Part model, mm, in its own coordinate system. Round coordinates to 2 decimals unless told otherwise and drop trailing zeros. Loops run counter-clockwise (first coordinate to the right, second up) from the corner with the lowest first, then second, coordinate; pieces in that order, holes last. Notation, with made-up numbers: (54.25, 18.5) -> (101.25, 18.5) arc R14 ccw to (101.25, 45.5) -> close; hole circle Ø8 at (57, -28.5). An arc over 180 degrees is marked (long way). Use a Markdown table: item, result. Add a question column.
Item 1: Flat gauge pin, fed straight in: pin 1 (15 mm diameter, centred on x = 437.11, z = -80.34, fed in from +Y) (1 decimal). Where does the tip first touch, or does it go through?
Item 2: Probe line 1 (X direction, y = 15.75, z = -48.5); line 2 (X direction, y = 4.5, z = -76.5). List the from-to ranges inside material, lowest first. Write a range as [from, to].
Item 3: Cut at C-C, the plane z = -82.5. List the corners of the cut face in (x, y), plus the area to 3 significant figures.
Item 4: Cut at B-B, the plane y = 10.5. List the corners of the cut face in (x, z), plus the area to 3 significant figures.
Item 5: Cut at A-A, the plane z = -37.5. List the corners of the cut face in (x, y).
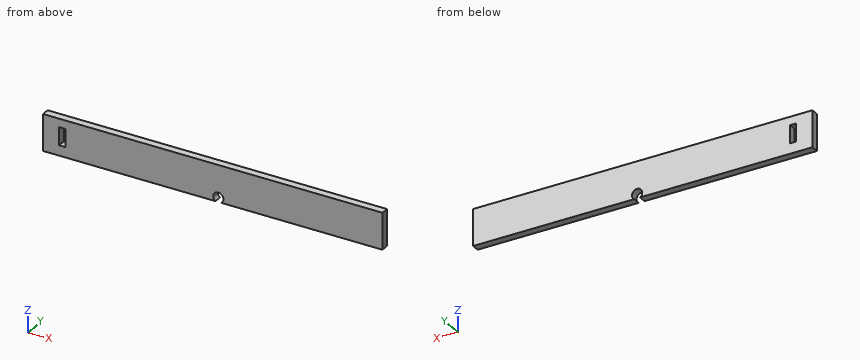
```python
from build123d import *

# Parameters (mm, degrees)
SKETCH1_W           = 846.328
SKETCH1_H           = 90.8304
BOSS_EXTRUDE1_DEPTH = 19.05
SKETCH2_R           = 12.7
CUT_EXTRUDE4_DEPTH  = 20.05
SKETCH4_W           = 15.156731747
SKETCH4_H           = 44.578622786
CUT_EXTRUDE5_DEPTH  = 20.05


with BuildPart() as part:
    # Sketch1 → Boss-Extrude1 (new body)
    with BuildSketch(Plane(origin=(0, 0, 0), x_dir=(1, 0, 0), z_dir=(0, 1, 0))):
        with Locations((423.164, 45.4152)):
            Rectangle(SKETCH1_W, SKETCH1_H)
    extrude(amount=BOSS_EXTRUDE1_DEPTH)

    # Sketch2 → Cut-Extrude4 (cut, through all)
    with BuildSketch(Plane.XZ):
        with Locations((437.1086, -80.3402)):
            Circle(SKETCH2_R)
    extrude(amount=-CUT_EXTRUDE4_DEPTH, mode=Mode.SUBTRACT)

    # Sketch4 → Cut-Extrude5 (cut, through all)
    with BuildSketch(Plane.XZ):
        with Locations((48.024327766, -43.050866134)):
            Rectangle(SKETCH4_W, SKETCH4_H)
    extrude(amount=-CUT_EXTRUDE5_DEPTH, mode=Mode.SUBTRACT)


solid = part.part
```
A:
| question | item | result |
|---|---|---|
| 1 | pin 1 | passes through |
| 2 | line 1 | x = [0, 40.45], [55.6, 846.33] |
| 2 | line 2 | x = [0, 425], [449.21, 846.33] |
| 3 | outline | (0, 0) -> (424.59, 0) -> (424.59, 19.05) -> (0, 19.05) -> close; (449.62, 0) -> (846.33, 0) -> (846.33, 19.05) -> (449.62, 19.05) -> close |
| 3 | area | 15,600 mm^2 |
| 4 | outline | (0, -90.83) -> (429.95, -90.83) arc R12.7 cw (long way) to (444.27, -90.83) -> (846.33, -90.83) -> (846.33, 0) -> (0, 0) -> close; hole (40.45, -65.34) -> (55.6, -65.34) -> (55.6, -20.76) -> (40.45, -20.76) -> close |
| 4 | area | 75,700 mm^2 |
| 5 | outline | (0, 0) -> (40.45, 0) -> (40.45, 19.05) -> (0, 19.05) -> close; (55.6, 0) -> (846.33, 0) -> (846.33, 19.05) -> (55.6, 19.05) -> close |
